Can you work these out from the model? Positions are in its coordinate system, mm. Face numbers are marked on the shaded views. A direction names the side the tool comes from. Round coordinates to 2 decimals unless told otherwise and drop trailing zeros. Write each loop counter-clockwise with the first axis right and the second up, starting at its lowest first coordinate (ties: lowest second). Pieces come first, ordered by that corner, then holes. Notation, with made-up numbers: (11.5, -7.5) -> (31.5, -7.5) arc R25 ccw to (31.5, 28.5) -> close; hole circle Ø9 at (4, 73). An arc over 180 degrees is marked (long way). Use CSV: the item, a comma, the result in double quotes.
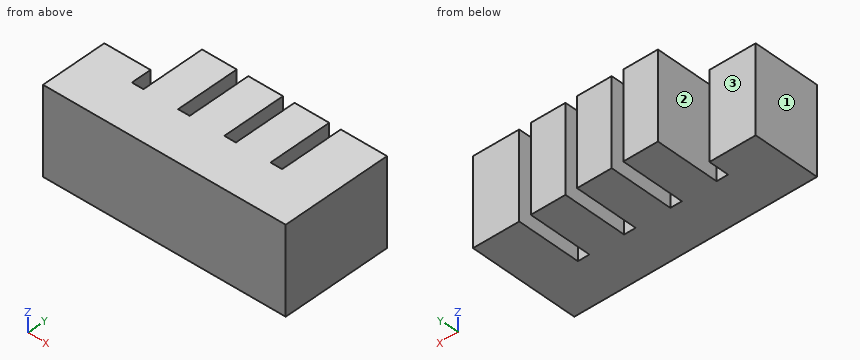
```python
from build123d import *

# Parameters (mm, degrees)
SKETCH1_W           = 6
SKETCH1_H           = 15
BOSS_EXTRUDE1_DEPTH = 15
SKETCH2_W           = 4
SKETCH2_H           = 11
CUT_EXTRUDE1_DEPTH  = 13
SKETCH3_W           = 15
SKETCH3_H           = 4
BOSS_EXTRUDE2_DEPTH = 2
LPATTERN1_COUNT     = 4
LPATTERN1_PITCH     = 8
SKETCH4_W           = 15
SKETCH4_H           = 15
BOSS_EXTRUDE3_DEPTH = 8
SKETCH5_W           = 4
SKETCH5_H           = 11
CUT_EXTRUDE2_DEPTH  = 5.5
SKETCH6_W           = 15
SKETCH6_H           = 15
BOSS_EXTRUDE4_DEPTH = 2
SKETCH7_W           = 36
SKETCH7_H           = 2
CUT_EXTRUDE3_DEPTH  = 2
SKETCH8_W           = 8
SKETCH8_H           = 15
CUT_EXTRUDE4_DEPTH  = 7.5
SKETCH9_W           = 42
SKETCH9_H           = 15
BOSS_EXTRUDE5_DEPTH = 4


with BuildPart() as part:
    # Sketch1 → Boss-Extrude1 (new body)
    with BuildSketch(Plane(origin=(0, 0, 0), x_dir=(1, 0, 0), z_dir=(0, 1, 0))):
        with Locations((3, 7.5)):
            Rectangle(SKETCH1_W, SKETCH1_H)
    extrude(amount=BOSS_EXTRUDE1_DEPTH)

    # Sketch2 → Cut-Extrude1 (cut)
    with BuildSketch(Plane.XZ):
        with Locations((3, -7.5)):
            Rectangle(SKETCH2_W, SKETCH2_H)
    extrude(amount=-CUT_EXTRUDE1_DEPTH, mode=Mode.SUBTRACT)

    # Sketch3 → Boss-Extrude2 (add)
    with BuildSketch(Plane.ZY):
        with Locations((-7.5, 2)):
            Rectangle(SKETCH3_W, SKETCH3_H)
    extrude(amount=BOSS_EXTRUDE2_DEPTH)


with BuildPart() as lpattern1_1:
    # LPattern1: pattern copy
    add(part.part.moved(Location(Vector(-1, 0, 0) * (1 * LPATTERN1_PITCH))))


with BuildPart() as lpattern1_2:
    # LPattern1: pattern copy
    add(part.part.moved(Location(Vector(-1, 0, 0) * (2 * LPATTERN1_PITCH))))


with BuildPart() as lpattern1_3:
    # LPattern1: pattern copy
    add(part.part.moved(Location(Vector(-1, 0, 0) * (3 * LPATTERN1_PITCH))))

    # Sketch4 → Boss-Extrude3 (add)
    with BuildSketch(Plane.ZY.offset(26)):
        with Locations((-7.5, 7.5)):
            Rectangle(SKETCH4_W, SKETCH4_H)
    extrude(amount=BOSS_EXTRUDE3_DEPTH)

    # Sketch5 → Cut-Extrude2 (cut)
    with BuildSketch(Plane.XZ):
        with Locations((-29, -7.5)):
            Rectangle(SKETCH5_W, SKETCH5_H)
    extrude(amount=-CUT_EXTRUDE2_DEPTH, mode=Mode.SUBTRACT)


with BuildPart() as lpattern1_1_1:
    add(lpattern1_1.part)

    # Combine1: union LPattern1_2, LPattern1_3, part
    add(lpattern1_2.part)
    add(lpattern1_3.part)
    add(part.part)

    # Sketch6 → Boss-Extrude4 (add)
    with BuildSketch(Plane(origin=(6, 0, 0), x_dir=(0, 0, -1), z_dir=(1, 0, 0))):
        with Locations((7.5, 7.5)):
            Rectangle(SKETCH6_W, SKETCH6_H)
    extrude(amount=BOSS_EXTRUDE4_DEPTH)

    # Sketch7 → Cut-Extrude3 (cut)
    with BuildSketch(Plane.XZ):
        with Locations((-13, -7.5)):
            Rectangle(SKETCH7_W, SKETCH7_H)
    extrude(amount=-CUT_EXTRUDE3_DEPTH, mode=Mode.SUBTRACT)

    # Sketch8 → Cut-Extrude4 (cut)
    with BuildSketch(Plane(origin=(0, 15, 0), x_dir=(1, 0, 0), z_dir=(0, 1, 0))):
        with Locations((-30, 7.5)):
            Rectangle(SKETCH8_W, SKETCH8_H)
    extrude(amount=-CUT_EXTRUDE4_DEPTH, mode=Mode.SUBTRACT)

    # Sketch9 → Boss-Extrude5 (add)
    with BuildSketch(Plane.XZ):
        with Locations((-13, -7.5)):
            Rectangle(SKETCH9_W, SKETCH9_H)
    extrude(amount=BOSS_EXTRUDE5_DEPTH)


solid = lpattern1_1_1.part
```
Q1. On a 3-axis mill with a long thin cutter (end or side, diameter ignored), from which of +Z, -Z, +X, -X, +Y, -Y can I reach the whole of each face in a straight line? I mean the marked faces 1, 2 and 3. Say none if no direction works.
Resolved:
face 1,"+Z, -Z, -X, +Y, -Y"
face 2,"+Z, -Z, +Y"
face 3,"+Z, -Z, -X, +Y"
Q2. Please list where these lines run through material, in increasing order: probe 1 along X at (y, z) = (1.75, -5.5); probe 2 along Z at (x, y) = (-13.5, 11.25); probe 3 along Y at (x, z) = (-12.5, -10.75).
Resolved:
probe 1,"x = -34 to -31, -27 to -23, -19 to -15, -11 to -7, -3 to 1, 5 to 8"
probe 2,"z = -15 to -13, -2 to 0"
probe 3,"y = -4 to 0, 13 to 15"
Q3. Will these pins go through, and if not, where does the flat tip stop? P1, Ø1.6, axis at x = -1, z = -4.5, coming from the +Y side; P2, Ø1.5, axis at y = 11, z = -7.5, coming from the -X side; P3, Ø4, axis at x = -31.5, z = -7, coming from the +Y side.
Resolved:
P1,"stops at y = 4"
P2,"stops at x = -24"
P3,"stops at y = 7.5"
Q4. Suppose I cut it at B-B (y = 2.5). Write out the boundary of the cut face in (x, z).
Resolved:
outline,"(-34, -15) -> (8, -15) -> (8, 0) -> (-34, 0) -> close; hole (-31, -13) -> (-27, -13) -> (-27, -2) -> (-31, -2) -> close; hole (-23, -13) -> (-19, -13) -> (-19, -2) -> (-23, -2) -> close; hole (-15, -13) -> (-11, -13) -> (-11, -2) -> (-15, -2) -> close; hole (-7, -13) -> (-3, -13) -> (-3, -2) -> (-7, -2) -> close; hole (1, -13) -> (5, -13) -> (5, -2) -> (1, -2) -> close"
Q5. Suppose I cut it at D-D (z = -13.5). Write out the boundary of the cut face in (x, y).
Resolved:
outline,"(-34, -4) -> (8, -4) -> (8, 15) -> (0, 15) -> (0, 4) -> (-2, 4) -> (-2, 15) -> (-8, 15) -> (-8, 4) -> (-10, 4) -> (-10, 15) -> (-16, 15) -> (-16, 4) -> (-18, 4) -> (-18, 15) -> (-24, 15) -> (-24, 4) -> (-26, 4) -> (-26, 7.5) -> (-34, 7.5) -> close"
Q6. Suppose I cut it at A-A (y = 12.5). Count the separate pieces of the cut face and the enclosed holes in it, and give its area (3 significant figures).
Resolved:
separate pieces,"4"
enclosed holes,"4"
area,"214 mm^2"
Q7. Suppose I cut it at C-C (x = -25). Write out the boundary of the cut face in (y, z).
Resolved:
outline,"(-4, -15) -> (4, -15) -> (4, 0) -> (-4, 0) -> close; hole (0, -8.5) -> (2, -8.5) -> (2, -6.5) -> (0, -6.5) -> close"
